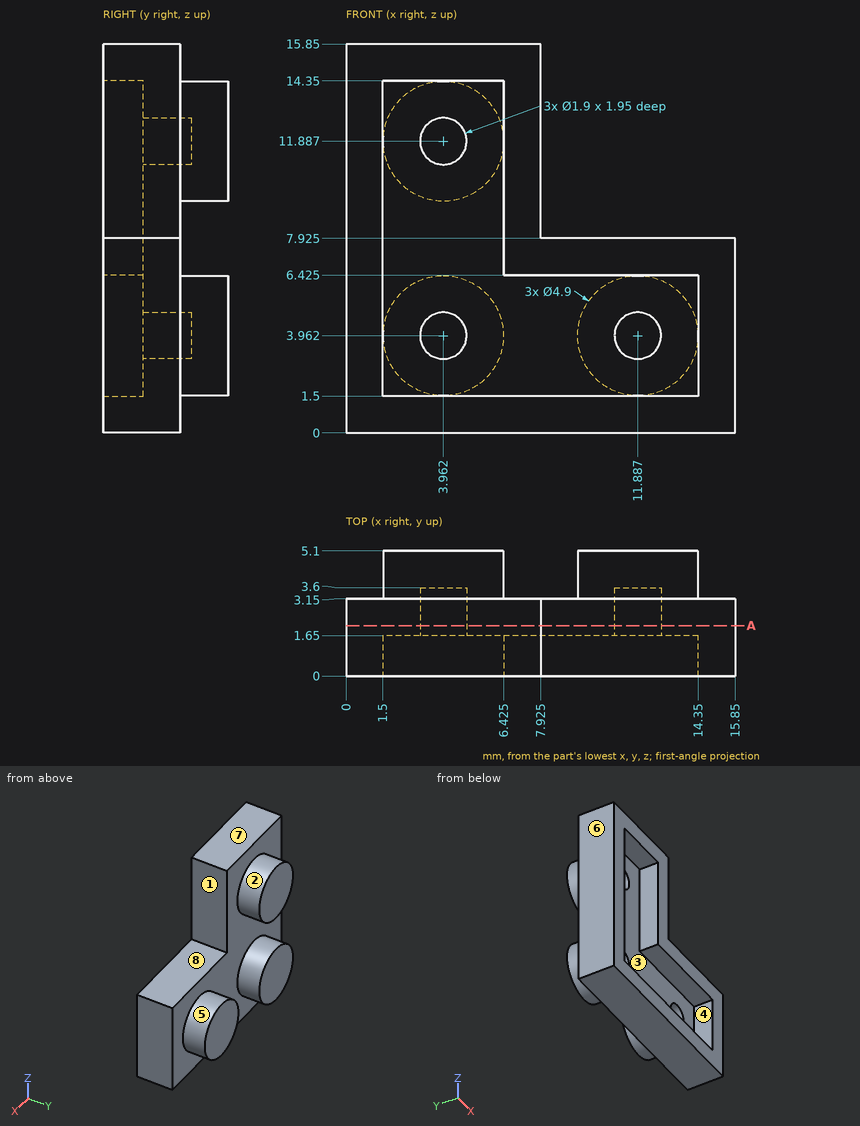
The figure shows three views and two pictorial views of one solid part (mm, origin at its lowest corner). Answer the questions. A direction names the side the tool comes from. Round coordinates to 2 decimals unless told otherwise and drop trailing zeros. Put each result on its own line as item: value. Start each with the question number.
Q1. For a pull along X with two mould halves and no side action, classify the marked faces 1, 2 and 3 as pulls with the +X half, pulls with the -X half, needs draft (parallel to the pull), parting line crosses it, or undercut.
Q2. A tool of negligible diameter and unlimited length cuts with its end or side. For the marked faces 4, 5, 6, 7 and 8, from which of +Z, -Z, +X, -X, +Y, -Y can it reach the whole face along a straight path? Write none if from no direction.
Q3. Flat-ended cylindrical pins translate along their axes: pin 1 (0.5 mm diameter, centred on x = 4.5, y = 0.5, fed in from -Z); pin 2 (1.7 mm diameter, centred on x = 3.96, z = 11.89, fed in from -Y); pin 3 (2 mm diameter, centred on x = 11.5, z = 4, fed in from -Y); pin 4 (0.5 mm diameter, centred on y = 1, z = 9, fed in from +X) (1 decimal). Find the tip coordinate at first contact, or state that the pin passes through.
Q4. Section A-A, the plane y = 2.05 is taken. Give the number of separate pieces and of enclosed holes in the cut face, and give its area (3 significant figures).
Q5. Straight lines are drawn through the part: L1, parallel to X at y = 0.55, z = 13.5 (1 decimal); L2, parallel to X at y = 0.9, z = 3.25; L3, parallel to Z at x = 13.5, y = 2.6 (1 decimal). For each, find the intervals that lie inside material, in ascending order. Write a range as [from, to].
Findings below:
1. face 1: pulls with the +X half
1. face 2: parting line crosses it
1. face 3: undercut
2. face 4: -Y
2. face 5: +Y
2. face 6: +Z, -Z, -X, +Y, -Y
2. face 7: +Z, +X, -X, +Y, -Y
2. face 8: +Z, +X, +Y, -Y
3. pin 1: stops at z = 0
3. pin 2: stops at y = 3.6
3. pin 3: stops at y = 1.65
3. pin 4: stops at x = 7.9
4. separate pieces: 1
4. enclosed holes: 3
4. area: 180 mm^2
5. L1: x = [0, 1.5], [6.4, 7.9]
5. L2: x = [0, 1.5], [14.35, 15.85]
5. L3: z = [0, 7.9]
